For this review, take the finished solid that the model builds, in its own axes (mm). A direction names the side the tool comes from. Coordinates: 2 decimals unless noted, no trailing zeros. Loops run counter-clockwise (first coordinate to the right, second up) from the corner with the lowest first, then second, coordinate; pieces in that order, holes last. Notation, with made-up numbers: (51.5, 16) -> (97.5, 16) arc R35 ccw to (97.5, 49) -> close; hole circle Ø1 at (-16, 18.5). An arc over 180 degrees is marked (long way). Answer in a Markdown table with one row per item.
from build123d import *

# Parameters (mm, degrees)
F0_W          = 5.5
F0_H          = 5.5
F0_W_2        = 2
F0_H_2        = 2
F1_DEPTH      = 15
F2_T          = -1
F3_START      = 3
F3_DEPTH      = 22
F5_DEPTH      = 16
F5_DEPTH_BACK = 3


with BuildPart() as f1:
    # F0 (on Top) → F1 (new body)
    with BuildSketch(Plane.XY):
        with Locations((3.75, 3.75)):
            Rectangle(F0_W, F0_H)
        with Locations((0, 3.75)):
            Rectangle(F0_W_2, F0_H)
        with Locations((-3.75, 3.75)):
            Rectangle(F0_W, F0_H)
        with Locations((-3.75, 0)):
            Rectangle(F0_W, F0_H_2)
        Rectangle(F0_W_2, F0_H_2)
        with Locations((3.75, 0)):
            Rectangle(F0_W, F0_H_2)
        with Locations((3.75, -3.75)):
            Rectangle(F0_W, F0_H)
        with Locations((0, -3.75)):
            Rectangle(F0_W_2, F0_H)
        with Locations((-3.75, -3.75)):
            Rectangle(F0_W, F0_H)
    extrude(amount=F1_DEPTH)

    # F2
    f2_openings = [f1.faces().sort_by_distance(p)[0] for p in [
        (0, 0, 15),
    ]]
    offset(amount=F2_T, openings=f2_openings)

    # F0 (on Top) → F3 (cut)
    with BuildSketch(Plane.XY.offset(F3_START)):
        with Locations((-3.75, 0)):
            Rectangle(F0_W, F0_H_2)
        with Locations((0, 3.75)):
            Rectangle(F0_W_2, F0_H)
        with Locations((3.75, 0)):
            Rectangle(F0_W, F0_H_2)
        with Locations((0, -3.75)):
            Rectangle(F0_W_2, F0_H)
    extrude(amount=F3_DEPTH, mode=Mode.SUBTRACT)

    # F4 (on face) → F5 (join, two sides)
    with BuildSketch(Plane.XZ.offset(6.5)) as f5_sk:
        Polygon((9.5, -2.5), (9.5, 0), (8.1, 0), (6.5, 0), (-6.5, 0), (-8.1, 0), (-9.5, 0), (-9.5, -2.5), align=None)
        with BuildLine():
            ThreePointArc((-8.1, 0), (-8.8, 0.7), (-9.5, 0))
            Line((-9.5, 0), (-8.1, 0))
        make_face()
        with BuildLine():
            Line((8.1, 0), (9.5, 0))
            ThreePointArc((9.5, 0), (8.8, 0.7), (8.1, 0))
        make_face()
        with BuildLine():
            add(Edge.make_bspline(
                [(-3.0857180245, -5.6900443979), (-2.6711979969, -5.6534883338), (-0.6382155364, -5.5259124188), (4.3516854172, -4.6654656415), (8.9744619057, -3.3519325688), (9.4804499148, -2.7164395318), (9.5, -2.5)],
                knots=[0.1581423577, 0.1581423577, 0.1581423577, 0.1581423577, 0.3379261215, 0.6272825134, 0.892948007, 1, 1, 1, 1], degree=3))
            Line((9.5, -2.5), (-9.5, -2.5))
            add(Edge.make_bspline(
                [(-3.4938230352, -5.7202531186), (-3.9193313832, -5.7494783037), (-4.8676868004, -5.791289792), (-6.2303397751, -5.5285607506), (-7.574736345, -4.9382947102), (-8.8313136046, -3.8354261533), (-9.278605125, -2.936326813), (-9.5, -2.5)],
                knots=[0.0502659739, 0.0502659739, 0.0502659739, 0.0502659739, 0.2077625312, 0.40408462, 0.5983848295, 0.8039601762, 1, 1, 1, 1], degree=3))
            add(Edge.make_bspline(
                [(-3.0857180245, -5.6900443979), (-3.2218733267, -5.7005172354), (-3.3580194857, -5.710925725), (-3.4938230352, -5.7202531186)],
                knots=[0, 0, 0, 0, 0.0502659739, 0.0502659739, 0.0502659739, 0.0502659739], degree=3))
        make_face()
    extrude(amount=-F5_DEPTH)
    extrude(f5_sk.sketch, amount=F5_DEPTH_BACK)


solid = f1.part
Item 1: Take a section at A-A, the plane z = 2. State the section outline as (x, y) points, and give its area (3 significant figures).
Worked answers:
| item | result |
|---|---|
| outline | (-6.5, -6.5) -> (6.5, -6.5) -> (6.5, 6.5) -> (-6.5, 6.5) -> close; hole (-5.5, -5.5) -> (5.5, -5.5) -> (5.5, 5.5) -> (-5.5, 5.5) -> close |
| area | 48.0 mm² |
Item 2: Insertion check: pin 1 (0.8 mm diameter, centred on x = -0.5, y = 6, fed in from +Z); pin 2 (10.5 mm diameter, centred on x = -1.5, z = 9, fed in from +Y); pin 3 (5 mm diameter, centred on y = 6.5, z = 9, fed in from +X). Each pin has a flat end and moves straight along its axis. Give the tip position at first contact, or say it passes through.
Worked answers:
| item | result |
|---|---|
| pin 1 | z = 3 |
| pin 2 | y = 6.5 |
| pin 3 | x = 6.5 |
Item 3: Take a section at B-B, the plane z = 13.75. State the section outline as (x, y) points.
Worked answers:
| item | result |
|---|---|
| outline | (-6.5, -6.5) -> (-1, -6.5) -> (-1, -5.5) -> (-5.5, -5.5) -> (-5.5, -1) -> (-6.5, -1) -> close; (-6.5, 1) -> (-5.5, 1) -> (-5.5, 5.5) -> (-1, 5.5) -> (-1, 6.5) -> (-6.5, 6.5) -> close; (1, -6.5) -> (6.5, -6.5) -> (6.5, -1) -> (5.5, -1) -> (5.5, -5.5) -> (1, -5.5) -> close; (1, 5.5) -> (5.5, 5.5) -> (5.5, 1) -> (6.5, 1) -> (6.5, 6.5) -> (1, 6.5) -> close |
Item 4: The part is to be moulded in two halves that separate along Y. For faces 1 (the flat face through (0, 6, 3)), 2 (the flat face through (6, 1, 9)), 3 (the flat face through (2, 6.5, 7)), say which applies: +Y half, -Y half, draft (parallel to the pull), parting line (faces both ways), or undercut.
Worked answers:
| item | result |
|---|---|
| face 1 | draft |
| face 2 | undercut |
| face 3 | +Y half |
Item 5: For L1, parallel to X at y = -4, z = 12.25; L2, parallel to X at y = 2.75, z = 0.5; L3, parallel to Y at x = -5.75, z = 6.25, list the stretches that pass through material, from the lowest coordinate up.
Worked answers:
| item | result |
|---|---|
| L1 | -6.5 to -5.5, 5.5 to 6.5 |
| L2 | -9.29 to -8.31, -6.5 to 6.5, 8.31 to 9.29 |
| L3 | -6.5 to -1, 1 to 6.5 |
Item 6: For faces 4 (the flat face through (-1.3, -5.5, 7.9)), 5 (the flat face through (6, -1, 9)), 6 (the flat face through (1, -6, 9)), list the 3-axis set-ups (+Z, -Z, +X, -X, +Y, -Y) from which the entire face can be reached by the end or side of a thin tool; tool diameter is ignored.
Worked answers:
| item | result |
|---|---|
| face 4 | +Z |
| face 5 | +Z, +X, -X |
| face 6 | +Z, +Y, -Y |
